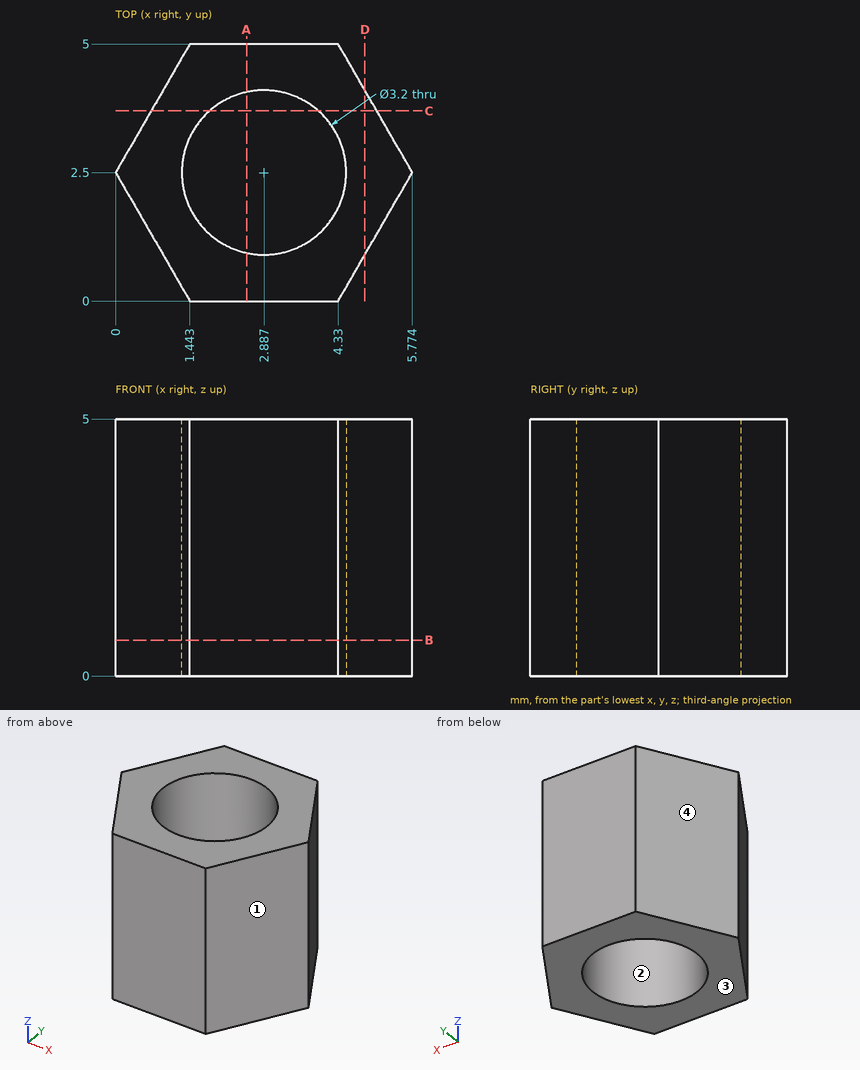
Print and shaded views of the part. All mm, measured from the part's lowest x, y and z. Give positions to 0.01 mm unless a question says otherwise; leave off trailing zeros. Loops run counter-clockwise (first coordinate to the right, second up) from the corner with the lowest first, then second, coordinate; pieces in that order, holes last.
1) Flat gauge pins, fed straight in: pin 1 Ø2 at (x, y) = (3.5, 1.5) entering from +Z; pin 2 Ø1.5 at (y, z) = (3.5, 4.5) entering from -X (1 decimal). Where does each tip first touch, or does it go through?
2) Saw through at D-D (x = 4.85). Write the cut outline in (y, z), plus the area to 3 significant figures.
3) Saw through at A-A (x = 2.55). Write the cut outline in (y, z) (1 decimal).
4) Saw through at B-B (z = 0.7). Write the cut outline in (x, y).
5) Pull direction Y, two halves, no side cores. Call the marked faces 1, 2, 3 and 4: +Y half, -Y half, draft (parallel to the pull), parting line (faces both ways), or undercut.
6) Saw through at C-C (y = 3.7). Write the cut outline in (x, z) (1 decimal).
7) Wall check: line 1 (Y direction, x = 4, z = 2.45); line 2 (Y direction, x = 3.7, z = 2.1); line 3 (X direction, y = 2.45, z = 0.55) (1 decimal). Give the ranges that are in metal, low to high.
Answer block:
1. pin 1: stops at z = 5
1. pin 2: stops at x = 0.1
2. outline: (0.9, 0) - (4.1, 0) - (4.1, 5) - (0.9, 5) - close
2. area: 16.0 mm2
3. outline: (0, 0) - (0.9, 0) - (0.9, 5) - (0, 5) - close; (4.1, 0) - (5, 0) - (5, 5) - (4.1, 5) - close
4. outline: (0, 2.5) - (1.44, 0) - (4.33, 0) - (5.77, 2.5) - (4.33, 5) - (1.44, 5) - close; hole circle Ø3.2 at (2.89, 2.5)
5. face 1: -Y half
5. face 2: undercut
5. face 3: draft
5. face 4: +Y half
6. outline: (0.7, 0) - (1.8, 0) - (1.8, 5) - (0.7, 5) - close; (3.9, 0) - (5.1, 0) - (5.1, 5) - (3.9, 5) - close
7. line 1: y = 0 to 1.35, 3.65 to 5
7. line 2: y = 0 to 1.12, 3.88 to 5
7. line 3: x = 0 to 1.3, 4.5 to 5.7
